Here's how the part is built. I have some questions about the finished solid (model axes, mm). A direction names the side the tool comes from. Coordinates: 2 decimals unless noted, no trailing zeros. Write each loop counter-clockwise with the first axis right and the second up, starting at its lowest first coordinate (ties: lowest second). Pieces come first, ordered by that corner, then holes. Notation, with made-up numbers: (81.25, 77.25) -> (108.25, 77.25) arc R32 ccw to (108.25, 108.25) -> close; hole circle Ø7 at (34.25, 46.5). An arc over 180 degrees is marked (long way). Use a Markdown table: item, result. Add a question column.
Item 1: If I drill on line 1 along Y through (x, z) = (-8.5, -4.25); line 2 along Z through (x, y) = (-3.5, 66.5); line 3 along Z through (x, y) = (-6, 70), over which ranges is the centre line in solid material (lowest first)? Write a range as from..to.
Item 2: Imagine slicing it at B-B, the plane x = -6.5. Write out the boundary of the cut face in (y, z).
Item 3: If we mould it in two halves opening along X, with no side actions, what happens to faces 3 (the cylindrical face through (-68.061, 75.093, 0.394)), 4 (the cylindrical face through (-3.659, 71.242, -5.354)), 5 (the cylindrical face through (-53.969, 75.261, -6.735))? For each: pulls with the +X half, pulls with the -X half, needs draft (parallel to the pull), parting line crosses it, or undercut.
Item 4: On a 3-axis mill with a long thin cutter (end or side, diameter ignored), from which of +Z, -Z, +X, -X, +Y, -Y can I reach the whole of each face in a straight line? I mean faces 1 (the cylindrical face through (-45.582, 72.436, 0.196)), 2 (the cylindrical face through (2.12, 71.24, 0.88)). Say none if no direction works.
Item 5: Will these pins go through, and if not, where does the flat tip stop? pin 1 Ø5 at (x, z) = (-46.5, -4) entering from -Y; pin 2 Ø5 at (y, z) = (52.5, -8) entering from +X; pin 3 Ø1 at (x, y) = (-61, 77.5) entering from +Z; pin 4 Ø1.5 at (x, y) = (-69.5, 52.5) entering from -Z.
Item 6: Imagine slicing it at A-A, the plane y = 95.5. Write out the boundary of the cut face in (x, z).
Autodesk Inventor part; units mm, degrees
ref_plane "作業平面1" through (-121.5758, 135, -17.9326) normal (0.516, 0, -0.8566) x (0.8566, 0, 0.516)
ref_plane "YZ Plane" through (0, 0, 0) normal (1, 0, 0) x (0, 1, 0)
ref_plane "XZ Plane" through (0, 0, 0) normal (0, 1, 0) x (-1, 0, 0)
sketch "スケッチ1" plane through (0, 0, 0) normal (0, 1, 0) x (-1, 0, 0)
  circle A0 centre (56.6667, -3.3333) radius 2
  circle A1 centre (6.6667, -1.3333) radius 2
  arc A2 (27.618, -9.313) -> (80.2911, 0.2239) centre (24.5838, 157.671) ccw
  arc A3 (20.5062, -9.2317) -> (27.618, -9.313) centre (25.435, 110.8283) ccw
  arc A4 (7.5483, -6.9284) -> (20.5062, -9.2317) centre (22.5133, 39.66) ccw
  arc A5 (0.14, -3.2897) -> (7.5483, -6.9284) centre (16.2383, 20.125) ccw
  arc A6 (-1.8521, -1.3552) -> (0.14, -3.2897) centre (4.8333, 3.5367) ccw
  arc A7 (-0.4054, 2.2589) -> (-1.8521, -1.3552) centre (0, 0) ccw
  arc A8 (5.081, 2.7563) -> (-0.4054, 2.2589) centre (5.1833, -28.88) ccw
  arc A9 (23.6457, 1.9287) -> (5.081, 2.7563) centre (5.71, -191.7767) ccw
  arc A10 (23.6457, 1.9287) -> (35.0642, 0.89) centre (351.2983, 3540.5833) ccw
  arc A11 (35.0642, 0.89) -> (56.4197, -0.0064) centre (55.24, 226.7233) ccw
  arc A12 (56.4197, -0.0064) -> (79.9865, 1.514) centre (55.3817, 199.4967) ccw
  arc A13 (80.2911, 0.2239) -> (79.9865, 1.514) centre (80.0687, 0.8524) ccw
extrude "押し出し1" add sketch "スケッチ1" along normal mid plane 250 contours A0 | A1 | A3 A4 A5 A6 A7 A8 A9 A10 A11 A12 A13 A2
ref_plane "作業平面1" through (-121.5758, 135, -17.9326) normal (0.516, 0, -0.8566) x (0.8566, 0, 0.516)
sketch "スケッチ4" plane through (-121.5758, 135, -17.9326) normal (0.516, 0, -0.8566) x (0.8566, 0, 0.516)
  arc A0 (90, 35) -> (0, 0) centre (90, -98.2143) ccw
  line L0 (183.3333, 35) -> (90, 35)
  line L1 (183.3333, 35) -> (183.3333, 0)
  line L2 (183.3333, 0) -> (0, 0)
  point P0 (113.3913, 135)
extrude "押し出し4" cut sketch "スケッチ4" along normal through all
sketch "スケッチ5" plane through (0, 0, 0) normal (1, 0, 0) x (0, 1, 0)
  line L0 (0, 23.0117) -> (-125, 23.0117)
  line L1 (-125, 23.0117) -> (-125, -26.2227)
  line L2 (-125, -26.2227) -> (0, -26.2227)
  line L3 (0, -26.2227) -> (0, 23.0117)
  line L4 (-125, 0.2239) -> (-125, -9.313)
  line L5 (-125, -9.313) -> (-125, -9.2317)
  line L6 (-125, -9.2317) -> (-125, -6.9284)
  line L7 (-125, -6.9284) -> (-125, -3.2897)
  line L8 (-125, -3.2897) -> (-125, -1.3552)
  line L9 (-125, -1.3552) -> (-125, 2.2589)
  line L10 (-125, 2.2589) -> (-125, 2.7563)
  line L11 (-125, 2.7563) -> (-125, 1.9287)
  line L12 (-125, 1.9287) -> (-125, 0.89)
  line L13 (-125, 0.89) -> (-125, -0.0064)
  line L14 (-125, -0.0064) -> (-125, 1.514)
  line L15 (-125, 1.514) -> (-125, 0.2239)
  line L16 (0, -36.0696) -> (0, 32.8586)
  point P0 (0, 0)
extrude "押し出し5" cut sketch "スケッチ5" along normal through all both and the other way through all
sketch "スケッチ6" plane through (0, 0, 0) normal (0, 1, 0) x (-1, 0, 0)
  circle A0 centre (5.6309, -1.5008) radius 3.25
  circle A1 centre (43.5535, -3.9243) radius 3.25
  point P0 (0, 0)
extrude "押し出し6" cut sketch "スケッチ6" along normal through all
sketch "スケッチ7" plane through (0, 0, 0) normal (1, 0, 0) x (0, 1, 0)
  line L0 (0, -4.7508) -> (0, 1.7492)
  line L1 (0, -7.1743) -> (0, -0.6743)
  line L2 (0, 0.89) -> (0, 1.9287)
  line L3 (0, -0.0064) -> (0, 0.89)
  line L4 (0, 1.514) -> (0, -0.0064)
  line L5 (0, 0.2239) -> (0, 1.514)
  line L6 (0, -9.313) -> (0, 0.2239)
  line L7 (0, -9.2317) -> (0, -9.313)
  line L8 (0, -6.9284) -> (0, -9.2317)
  line L9 (0, -3.2897) -> (0, -6.9284)
  line L10 (0, -1.3552) -> (0, -3.2897)
  line L11 (0, 2.2589) -> (0, -1.3552)
  line L12 (0, 2.7563) -> (0, 2.2589)
  line L13 (0, 1.9287) -> (0, 2.7563)
  line L14 (0, 35.5513) -> (41.667, 35.5513)
  line L15 (41.667, 35.5513) -> (41.667, -19.8637)
  line L16 (41.667, -19.8637) -> (0, -19.8637)
  line L17 (0, -19.8637) -> (0, 35.5513)
  point P0 (0, 0)
  dimension "d19" = 41.667
extrude "押し出し7" cut sketch "スケッチ7" along normal through all both and the other way through all
properties part number "newsubflap_top"
Ans:
| question | item | result |
|---|---|---|
| 1 | line 1 | y = 41.67..100 |
| 1 | line 2 | z = -5.27..-3.95, 0.95..2.71 |
| 1 | line 3 | z = -6.38..-4.73, 1.73..2.76 |
| 2 | outline | (41.67, -6.57) -> (100, -6.57) -> (100, -4.63) -> (41.67, -4.63) -> close; (41.67, 1.63) -> (100, 1.63) -> (100, 2.76) -> (41.67, 2.76) -> close |
| 3 | face 3 | undercut |
| 3 | face 4 | pulls with the +X half |
| 3 | face 5 | pulls with the -X half |
| 4 | face 1 | +Z, +Y, -Y |
| 4 | face 2 | +X, +Y, -Y |
| 5 | pin 1 | stops at y = 41.67 |
| 5 | pin 2 | stops at x = -3.96 |
| 5 | pin 3 | stops at z = 0.08 |
| 5 | pin 4 | stops at z = -3.39 |
| 6 | outline | (-80.29, 0.22) arc R167.02 ccw to (-27.62, -9.31) arc R120.16 ccw to (-20.51, -9.23) arc R48.93 ccw to (-7.55, -6.93) arc R28.41 ccw to (-0.14, -3.29) arc R8.29 ccw to (1.85, -1.36) arc R2.29 ccw to (0.41, 2.26) arc R31.63 ccw to (-5.08, 2.76) arc R194.55 ccw to (-23.65, 1.93) arc R3557.02 cw to (-35.06, 0.89) arc R226.74 cw to (-56.42, -0.01) arc R199.49 cw to (-79.99, 1.51) arc R0.67 ccw to start; hole circle Ø6.5 at (-43.55, -3.92); hole circle Ø6.5 at (-5.63, -1.5) |
